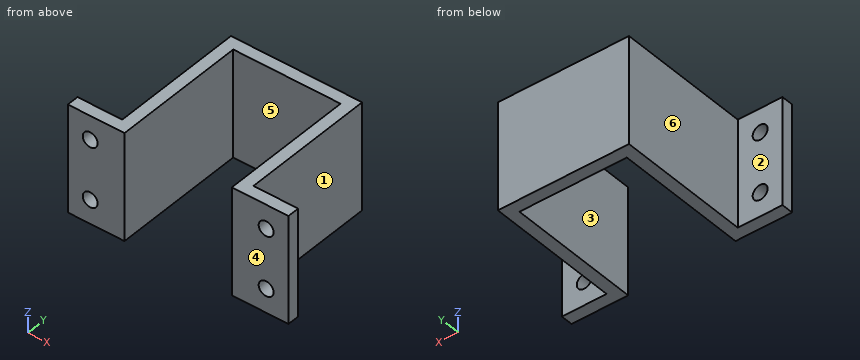
from build123d import *

# Parameters (mm, degrees)
EXTRUDE_1_DEPTH     = 36
SKETCH_2_R          = 2.5
CUT_EXTRUDE_1_DEPTH = 36


with BuildPart() as part:
    # 草图1 → 凸台-拉伸1 (new body)
    with BuildSketch(Plane.XY):
        Polygon((-4, 0), (0, 0), (36, 0), (40, 0), (40, -45), (55, -45), (55, -49), (40, -49), (36, -49), (36, -4), (0, -4), (0, -49), (-4, -49), (-19, -49), (-19, -45), (-4, -45), align=None)
    extrude(amount=EXTRUDE_1_DEPTH)

    # 草图2 → 切除-拉伸1 (cut)
    with BuildSketch(Plane(origin=(0, -45, 0), x_dir=(1, 0, 0), z_dir=(0, 1, 0))):
        with Locations(Location((-11.5, -8, 0), (0, 0, 270))):
            Circle(SKETCH_2_R)
        with Locations(Location((-11.5, -28, 0), (0, 0, 270))):
            Circle(SKETCH_2_R)
        with Locations(Location((47.5, -28, 0), (0, 0, 270))):
            Circle(SKETCH_2_R)
        with Locations(Location((47.5, -8, 0), (0, 0, 270))):
            Circle(SKETCH_2_R)
    extrude(amount=-CUT_EXTRUDE_1_DEPTH, mode=Mode.SUBTRACT)


solid = part.part
Build history of the part. All positions in model axes, mm. Face numbers are marked on the shaded views. A direction names the side the tool comes from. Round coordinates to 2 decimals unless told otherwise and drop trailing zeros. Loops run counter-clockwise (first coordinate to the right, second up) from the corner with the lowest first, then second, coordinate; pieces in that order, holes last. Notation, with made-up numbers: (13, 49.25) -> (46, 49.25) arc R17 cw to (46, 54.25) -> close; hole circle Ø10 at (63.5, -32.75). An arc over 180 degrees is marked (long way). One line per item, written item: value. Start each with the question number.
Q1. Drop flat-ended pins along their axis: pin 1 Ø1.5 at (x, z) = (32.5, 17.5) entering from +Y; pin 2 Ø4 at (y, z) = (-29.5, 25.5) entering from -X; pin 3 Ø18 at (y, z) = (-35.5, 13) entering from +X; pin 4 Ø8 at (x, z) = (22, 16) entering from -Y. Give the stop position or say it passes through.
Q2. Cut at A-A on y = -15. List the corners of the cut face in (x, z).
Q3. Two-plate mould, pull along X, no slides. Class the marked faces 4, 5 and 6: released by +X, released by -X, zero draft, split by the parting line, or undercut.
Q4. Cut at B-B on z = 8. List the corners of the cut face in (x, y), plus the area to 3 significant figures.
Q5. Cut at C-C on x = 47.5. List the corners of the cut face in (y, z), plus the area to 3 significant figures.
Q6. Probe line 1 along X through (y, z) = (-47, 8); line 2 along X through (y, z) = (-39, 28); line 3 along Z through (x, y) = (-11, -48). List the from-to ranges inside material, lowest first.
Q7. Cut at D-D on z = 17. List the corners of the cut face in (x, y), plus the area to 3 significant figures.
Q8. 3-axis set-ups, long thin cutter, end or side, ignore diameter. For the marked faces 1, 2 and 3: which of +Z, -Z, +X, -X, +Y, -Y reach the whole face in a straight line?
Computed:
1. pin 1: y = 0
1. pin 2: x = -4
1. pin 3: x = 40
1. pin 4: y = -4
2. outline: (-4, 0) -> (0, 0) -> (0, 36) -> (-4, 36) -> close; (36, 0) -> (40, 0) -> (40, 36) -> (36, 36) -> close
3. face 4: zero draft
3. face 5: undercut
3. face 6: released by -X
4. outline: (-19, -49) -> (-14, -49) -> (-14, -45) -> (-19, -45) -> close; (-9, -49) -> (0, -49) -> (0, -4) -> (36, -4) -> (36, -49) -> (45, -49) -> (45, -45) -> (40, -45) -> (40, 0) -> (-4, 0) -> (-4, -45) -> (-9, -45) -> close; (50, -49) -> (55, -49) -> (55, -45) -> (50, -45) -> close
4. area: 616 mm²
5. outline: (-49, 0) -> (-45, 0) -> (-45, 5.5) -> (-49, 5.5) -> close; (-49, 10.5) -> (-45, 10.5) -> (-45, 25.5) -> (-49, 25.5) -> close; (-49, 30.5) -> (-45, 30.5) -> (-45, 36) -> (-49, 36) -> close
5. area: 104 mm²
6. line 1: -19 to -14, -9 to 0, 36 to 45, 50 to 55
6. line 2: -4 to 0, 36 to 40
6. line 3: 0 to 5.55, 10.45 to 25.55, 30.45 to 36
7. outline: (-19, -49) -> (0, -49) -> (0, -4) -> (36, -4) -> (36, -49) -> (55, -49) -> (55, -45) -> (40, -45) -> (40, 0) -> (-4, 0) -> (-4, -45) -> (-19, -45) -> close
7. area: 656 mm²
8. face 1: +Z, -Z, +X, +Y
8. face 2: +Z, -Z, -X, +Y
8. face 3: +Z, -Z, -Y
